Autodesk Inventor part; units mm, degrees
ref_plane "YZ Plane" through (0, 0, 0) normal (1, 0, 0) x (0, 1, 0)
ref_plane "XZ Plane" through (0, 0, 0) normal (0, 1, 0) x (-1, 0, 0)
ref_plane "XY Plane" through (0, 0, 0) normal (0, 0, 1) x (1, 0, 0)
sketch "Sketch1" plane through (0, 0, 0) normal (0, 0, 1) x (1, 0, 0)
  circle A0 centre (2.5244, 2.0294) radius 10
  point P0 (0, 0)
  dimension "d0" = 20
extrude "Extrusion1" add sketch "Sketch1" along normal blind 3
sketch "Sketch2" plane through (2.5244, 2.0294, 3) normal (0, 0, 1) x (1, 0, 0)
  circle A0 centre (0, 0) radius 10
  circle A1 centre (0, 0) radius 7.5
  point P0 (-2.5244, -2.0294)
  dimension "d3" = 15
extrude "Extrusion2" add sketch "Sketch2" along normal blind 6.9
sketch "Sketch3" plane through (2.5244, 2.0294, 3) normal (0, 0, 1) x (1, 0, 0)
  circle A0 centre (0, 0) radius 7.5
  circle A1 centre (0, 0) radius 5.95
  arc A2 (-3.0017, 1.8) -> (3.0017, 1.8) centre (0, 0) ccw
  line L0 (0, 1.8) -> (3.0017, 1.8)
  line L1 (0, 1.8) -> (-3.0017, 1.8)
  line L2 (0, 1.8) -> (0, -3.5)
  point P0 (-2.5244, -2.0294)
  dimension "d6" = 11.9
  dimension "d7" = 7
  dimension "d18" = 5.3
extrude "Extrusion3" add sketch "Sketch3" along normal blind 6.9 contours A1
fillet "Fillet1" radius 2 1 edges at (-7.4756, 2.0294, 0)
sketch "Sketch4" plane through (2.5244, 2.0294, 0) normal (0, 0, -1) x (-1, 0, 0)
  circle A0 centre (0, 0) radius 8
  line L0 (-8, 0) -> (-7.9961, 0.25)
  line L1 (-7.9961, 0.25) -> (-7.9961, -0.25)
  line L2 (-7.9961, -0.25) -> (-9.9703, -0.25)
  line L3 (-9.9703, -0.25) -> (-9.9703, 0.25)
  line L4 (-9.9703, 0.25) -> (-7.9961, 0.25)
  point P0 (2.5244, -2.0294)
  dimension "d12" = 0.25
  dimension "d13" = 0.5
extrude "Extrusion4" add sketch "Sketch4" against normal blind 1.85 contours A0 L2 L3 L4
sketch "Sketch5" plane through (0, 0, 0) normal (0, 0, -1) x (-1, 0, 0)
  line L0 (-10.5205, 2.2794) -> (-12.4947, 2.2794)
  line L1 (-12.4947, 2.2794) -> (-10.5205, 2.2794)
  line L2 (-10.5205, 2.2794) -> (-10.5205, 1.7794)
  line L3 (-10.5205, 1.7794) -> (-12.4947, 1.7794)
  line L4 (-12.4947, 1.7794) -> (-12.4947, 2.2794)
  point P0 (0, 0)
extrude "Extrusion5" add sketch "Sketch5" along normal blind 0.35
sketch "Sketch7" plane through (2.5244, 2.0294, 9.9) normal (0, 0, 1) x (1, 0, 0)
  arc A0 (-3.0017, 1.8) -> (3.0017, 1.8) centre (0, 0) ccw
  line L0 (-3.0017, 1.8) -> (3.0017, 1.8)
  circle A1 centre (0, 0) radius 5.95
  line L1 (3.0017, 1.8) -> (3.0017, 3.9445)
  point P0 (-2.5244, -2.0294)
extrude "Extrusion6" add sketch "Sketch7" along normal blind 2
sketch "Sketch8" plane through (2.5244, 2.0294, 9.9) normal (0, 0, 1) x (1, 0, 0)
  circle A0 centre (0, 0) radius 7.5
  circle A1 centre (0, 0) radius 10
  circle A2 centre (0, 0) radius 7.5
  circle A3 centre (0, 0) radius 10
  point P0 (-2.5244, -2.0294)
extrude "Extrusion7" add sketch "Sketch8" along normal blind 2
properties part number "knob"
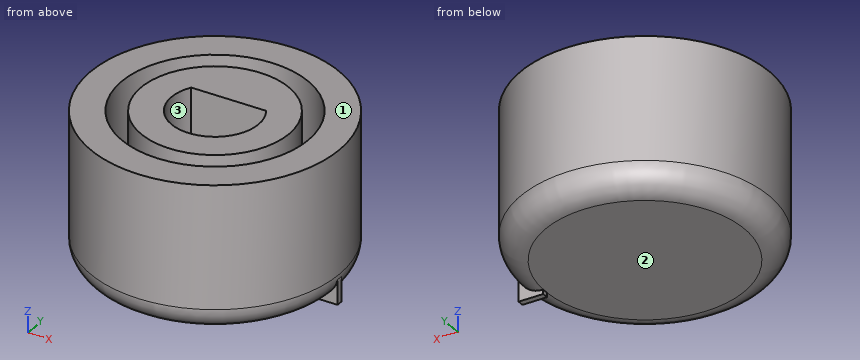
Part model, mm, in its own coordinate system. Face numbers are marked on the shaded views. A direction names the side the tool comes from. Give positions to 0.01 mm unless a question says otherwise; leave off trailing zeros. Write each loop counter-clockwise with the first axis right and the second up, starting at its lowest first coordinate (ties: lowest second). Pieces come first, ordered by that corner, then holes. Notation, with made-up numbers: (4, 4.5) -> (15, 4.5) arc R20 ccw to (15, 22.5) -> close; hole circle Ø7 at (6.25, 12). An arc over 180 degrees is marked (long way). Put each result on its own line as item: value. Start each with the question number.
Item 1: Which spindle directions (+Z, -Z, +X, -X, +Y, -Y) get a long thin tool onto all of the face, cutting with end or side? Do the marked faces 1, 2 and 3. Say none if no direction does.
Item 2: Wall check: L1, parallel to X at y = 4, z = 8.25; L2, parallel to Y at x = 2, z = 4.25; L3, parallel to X at y = 2.75, z = 10.25. Give the ranges that are in metal, low to high. Write a range as [from, to].
Item 3: Pin check, flat tips, straight feed: pin 1 Ø4 at (y, z) = (8, 3) entering from +X; pin 2 Ø3 at (x, z) = (-2, 6) entering from -Y; pin 3 Ø3 at (y, z) = (9.5, 7) entering from -X. Stop position of each tip, or through.
Item 4: Cut at A-A (z = 9). List the corners of the cut face in (x, y), then the cut area to 3 significant figures.
Answer list:
1. face 1: +Z, +X, -X, +Y, -Y
1. face 2: -Z, -X, +Y, -Y
1. face 3: +Z
2. L1: x = [-7.28, -4.71], [-3.09, 8.14], [9.76, 12.33]
2. L2: y = [-7.96, -5.45], [-3.9, -1.43], [3.83, 7.96], [9.51, 12.02]
2. L3: x = [-7.45, -4.94], [-3.38, -0.9], [5.95, 8.43], [9.99, 12.5]
3. pin 1: stops at x = 11.7
3. pin 2: stops at y = -7.5
3. pin 3: stops at x = -5.5
4. outline: circle Ø20 at (2.52, 2.03); circle Ø11.9 at (2.52, 2.03); hole circle Ø15 at (2.52, 2.03); hole (-0.48, 3.83) arc R3.5 ccw (long way) to (5.53, 3.83) -> close
4. area: 217 mm2
